Could you check a few things on this model? Use its own coordinates, in mm. Face numbers are marked on the shaded views. Round coordinates to 2 decimals unless told otherwise and drop trailing zeros. Order: outer loops, then holes, each group sorted by start corner. A loop starts at its lowest first (then second) coordinate and runs counter-clockwise, first axis right, second up. Notation, with made-up numbers: (-36.75, -7.5) -> (-25.75, -7.5) arc R14 ccw to (-25.75, -1.5) -> close; hole circle Ø3 at (30.5, 47). An arc over 180 degrees is marked (long way). One line per question, with ' | ' between items.
```python
from build123d import *

# Parameters (mm, degrees)
SKETCH1_W           = 25
SKETCH1_H           = 10
BOSS_EXTRUDE1_DEPTH = 9.5
CHAMFER1_SIZE       = 9
SKETCH3_W           = 16
SKETCH3_H           = 2
CUT_EXTRUDE2_DEPTH  = 3
SKETCH4_R           = 1.25
CUT_EXTRUDE3_DEPTH  = 4


with BuildPart() as part:
    # Sketch1 → Boss-Extrude1 (new body)
    with BuildSketch(Plane(origin=(0, 0, 0), x_dir=(1, 0, 0), z_dir=(0, 1, 0))):
        Rectangle(SKETCH1_W, SKETCH1_H)
    extrude(amount=BOSS_EXTRUDE1_DEPTH)

    # Chamfer1
    chamfer1_edges = [part.edges().sort_by_distance(p)[0] for p in [
        (-12.5, 9.5, 0),
    ]]
    chamfer(chamfer1_edges, length=CHAMFER1_SIZE)

    # Sketch3 → Cut-Extrude2 (cut)
    with BuildSketch(Plane(origin=(0, 9.5, 0), x_dir=(1, 0, 0), z_dir=(0, 1, 0))):
        with Locations((4.5, 2)):
            Rectangle(SKETCH3_W, SKETCH3_H)
        with Locations((4.5, -2)):
            Rectangle(SKETCH3_W, SKETCH3_H)
    extrude(amount=-CUT_EXTRUDE2_DEPTH, mode=Mode.SUBTRACT)

    # Sketch4 → Cut-Extrude3 (cut)
    with BuildSketch(Plane(origin=(-6.5, 6.5, 0), x_dir=(0, 0, 1), z_dir=(-0.707106781, 0.707106781, 0))):
        with Locations((0, 1.392640687)):
            Circle(SKETCH4_R)
    extrude(amount=-CUT_EXTRUDE3_DEPTH, mode=Mode.SUBTRACT)


solid = part.part
```
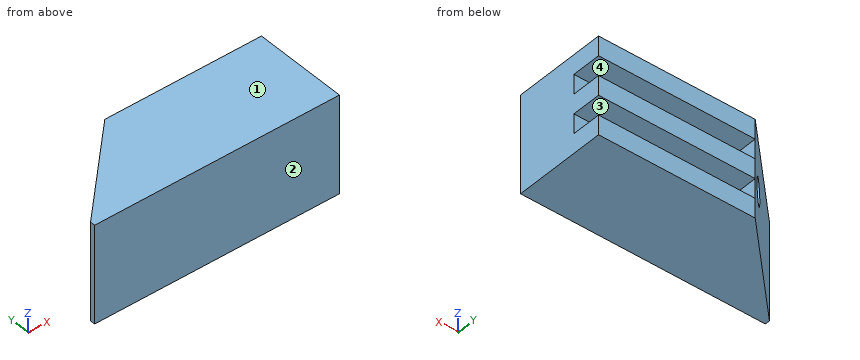
1. I want a section at B-B on x = 3.25. List the corners of the cut face in (y, z) for me, and give its area (3 significant figures).
From the geometry:
outline: (0, -5) -> (9.5, -5) -> (9.5, -3) -> (6.5, -3) -> (6.5, -1) -> (9.5, -1) -> (9.5, 1) -> (6.5, 1) -> (6.5, 3) -> (9.5, 3) -> (9.5, 5) -> (0, 5) -> close | area: 83.0 mm²
2. I want a section at D-D on y = 3. List the corners of the cut face in (x, z) for me, and give its area (3 significant figures).
From the geometry:
outline: (-10, -5) -> (12.5, -5) -> (12.5, 5) -> (-10, 5) -> close | area: 225 mm²
3. I want a section at C-C on z = 1.5. List the corners of the cut face in (x, y) for me, and give its area (3 significant figures).
From the geometry:
outline: (-12.5, 0) -> (12.5, 0) -> (12.5, 6.5) -> (-3.5, 6.5) -> (-3.5, 9.5) -> (-12.5, 0.5) -> close | area: 149 mm²
4. I want a section at A-A on y = 8.75. List the corners of the cut face in (x, z) for me, and give its area (4 significant figures).
From the geometry:
outline: (-4.25, -5) -> (12.5, -5) -> (12.5, -3) -> (-3.5, -3) -> (-3.5, -1) -> (12.5, -1) -> (12.5, 1) -> (-3.5, 1) -> (-3.5, 3) -> (12.5, 3) -> (12.5, 5) -> (-4.25, 5) -> close | area: 103.5 mm²
5. I'm going to push flat-ended pins straight in: pin 1 (2 mm diameter, centred on y = 3.5, z = -2.5, fed in from -X); pin 2 (0.6 mm diameter, centred on y = 7.5, z = 2, fed in from +X). Where does each tip first touch, or does it pass through?
From the geometry:
pin 1: stops at x = -10.5 | pin 2: stops at x = -3.5
6. I need wall thicknesses on probe 1 along Z at (x, y) = (0.75, 8.75); probe 2 along Y at (x, z) = (-2.25, -2.5); probe 3 along X at (y, z) = (5.5, -0.5). Which ranges of each line are inside material? Lowest first, please.
From the geometry:
probe 1: z = -5 to -3, -1 to 1, 3 to 5 | probe 2: y = 0 to 6.5 | probe 3: x = -7.5 to -5.15, -1.91 to 12.5
7. If we mould it in two halves opening along Z, with no side actions, what happens to the marked faces 1, 2, 3 and 4? For each: pulls with the +Z half, pulls with the -Z half, needs draft (parallel to the pull), parting line crosses it, or undercut.
From the geometry:
face 1: pulls with the +Z half | face 2: needs draft | face 3: undercut | face 4: undercut
